```python
from build123d import *

# Parameters (mm, degrees)
SKETCH2_R          = 7.5
SWEEP2_START       = -58
SWEEP2_OUTLINE_R   = 7.5
SWEEP2_DEPTH       = 45
SWEEP2_2_OUTLINE_R = 7.5
SWEEP2_2_ANGLE     = 90


with BuildPart() as part:
    # Sweep1: sweep along a path in Sketch1
    with BuildLine(Plane(origin=(0, 0, 0), x_dir=(0, 0, -1), z_dir=(1, 0, 0))) as sweep1_path:
        Line((-125, 265), (-82.266183324, 225.150071262))
        ThreePointArc((-82.266183324, 225.150071262), (-65.661209715, 205.006627523), (-54.835543734, 181.251871572))
        Line((-54.835543734, 181.251871572), (-34.369524404, 114.310538655))
        ThreePointArc((-34.369524404, 114.310538655), (-31.098413664, 99.854309295), (-30, 85.073368182))
        Line((-30, 85.073368182), (-30, 10))
        ThreePointArc((-30, 10), (-27.071067812, 2.928932188), (-20, 0))
        Line((-20, 0), (0, 0))
    # Sketch2 → Sweep1 (sweep)
    with BuildSketch(Plane.XY):
        Circle(SKETCH2_R)
    sweep(path=sweep1_path.line)

    # Sketch3 → Revolve1 (revolve)
    with BuildSketch(Plane(origin=(0, 0, 0), x_dir=(0, 0, -1), z_dir=(1, 0, 0))):
        with BuildLine():
            Line((-146.940611049, 285.459950802), (-125, 265))
            Line((-125, 265), (-118.521015579, 271.947860165))
            Line((-118.521015579, 271.947860165), (-133.977346338, 293.118807582))
            Line((-133.977346338, 293.118807582), (-134.213781062, 293.442658514))
            add(Edge.make_bspline(
                [(-134.213781062, 293.442658514), (-137.039454328, 296.077641462), (-146.940611049, 285.459950802)],
                knots=[3.152090242, 3.152090242, 3.152090242, 4.71238898, 4.71238898, 4.71238898], degree=2, weights=[0.958581046, 0.692308113, 1]))
        make_face()
    revolve(axis=Axis((0, 265, 125), (0, 0.6819983600624947, 0.731353701619174)))



with BuildPart() as body_2:
    # Sweep2: read off the stored shape, not the designer's step
    # Sweep2 outline → Sweep2 (new body)
    with BuildSketch(Plane.YZ.offset(SWEEP2_START)):
        with Locations((0, -13)):
            Circle(SWEEP2_OUTLINE_R)
    extrude(amount=SWEEP2_DEPTH)


with BuildPart() as part_1:
    add(part.part)

    add(body_2.part)  # Sweep2 2 merges body 2
    # Sweep2 2 outline → Sweep2 2 (revolve)
    with BuildSketch(Plane(origin=(-13, 0, 0), x_dir=(1, 0, 0), z_dir=(0, 0, 1))):
        with Locations((13, 0)):
            Circle(SWEEP2_2_OUTLINE_R)
    revolve(axis=Axis((-13, 0, 0), (0, 1, 0)), revolution_arc=SWEEP2_2_ANGLE)

    # Sketch6 → Revolve2 (revolve)
    with BuildSketch(Plane(origin=(0, 0, 0), x_dir=(1, 0, 0), z_dir=(0, 1, 0)), mode=Mode.PRIVATE) as revolve2_sk:
        with BuildLine():
            Line((-58, 33), (-58, 13))
            Line((-58, 13), (-25, 13))
            Line((-25, 13), (-25, 20.5))
            Line((-25, 20.5), (-19.159518744, 20.5))
            Line((-19.159518744, 20.5), (-25.39084721, 31.480649088))
            ThreePointArc((-25.39084721, 31.480649088), (-26.490355549, 32.592484066), (-28, 33))
            Line((-28, 33), (-58, 33))
        make_face()
        Polygon((-65, 13), (-58, 13), (-58, 33), (-58, 43), (-65, 43), align=None)
    revolve(revolve2_sk.sketch.rotate(Axis((-58, 0, -13), (1, 0, 0)), 180), axis=Axis((-58, 0, -13), (1, 0, 0)))


solid = part_1.part
```
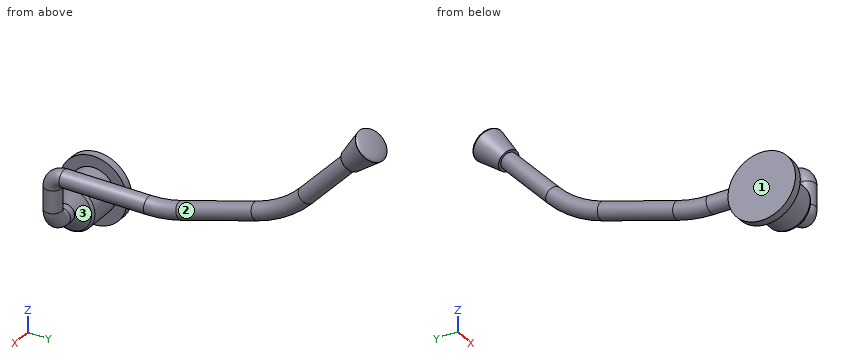
Check sheet for the modelled part. Datum: model origin and axes. Units: mm. Face numbers are marked on the shaded views. Give positions to 0.01 mm unless a question says otherwise; leave off trailing zeros. Loops run counter-clockwise (first coordinate to the right, second up) from the corner with the lowest first, then second, coordinate; pieces in that order, holes last. Notation, with made-up numbers: M 65.5,-11.75 L 74.5,-11.75 A27 cw 74.5,5.25 Z; hole C 68,16 d7. An arc over 180 degrees is marked long. Answer as CSV lines item,"result".
Item 1: Draft check along X on the marked faces 1, 2 and 3. Enter one of: pulls with the +X half, pulls with the -X half, needs draft (parallel to the pull), parting line crosses it, or undercut.
Reply:
face 1,"pulls with the -X half"
face 2,"parting line crosses it"
face 3,"undercut"
Item 2: Sectioned sample at A-A, the plane x = -51. Enter the section's corners in (y, z), then the cut area to 3 significant figures.
Reply:
outline,"C 0,-13 d40"
area,"1,260 mm^2"
Item 3: Scan lines: L1, parallel to Z at x = 4, y = 8; L2, parallel to Y at x = 9, z = 145; L3, parallel to Y at x = 3, z = 2. Record each from-to range of solid material in increasing order.
Reply:
L1,"23.06 to 36.22"
L2,"270.72 to 286.26"
L3,"-6.87 to 6.87"
Item 4: Depth check by flat-ended pin: pin 1 Ø12 at (y, z) = (228.5, 79) entering from -X. Enter the tip coordinate at first touch or a pass-through.
Reply:
pin 1,"x = -7.5"
